from build123d import *

# Parameters (mm, degrees)
BOSS_EXTRUDE1_DEPTH = 3.175
SKETCH2_W           = 3.175
SKETCH2_H           = 6.992
SKETCH2_W_2         = 12.5
SKETCH2_H_2         = 3.175
SKETCH2_W_3         = 15
CUT_EXTRUDE1_DEPTH  = 4.1750001


with BuildPart() as part:
    # Sketch1 → Boss-Extrude1 (new body)
    with BuildSketch(Plane(origin=(0, 0, 0), x_dir=(1, 0, 0), z_dir=(0, 1, 0))):
        with BuildLine():
            add(Edge.make_bspline(
                [(0, 0), (2.315309036, 13.13077004), (22.407654518, 25), (42.5, 25)],
                knots=[0, 0, 0, 0, 0.5, 0.5, 0.5, 0.5], degree=3))
            Line((0, 0), (42.5, 0))
            Line((42.5, 0), (42.5, 25))
        make_face()
        with BuildLine():
            Line((42.5, 25), (42.5, 0))
            Line((42.5, 0), (85, 0))
            add(Edge.make_bspline(
                [(42.5, 25), (62.592345482, 25), (82.684690964, 13.13077004), (85, 0)],
                knots=[0.5, 0.5, 0.5, 0.5, 1, 1, 1, 1], degree=3))
        make_face()
    extrude(amount=BOSS_EXTRUDE1_DEPTH)

    # Sketch2 → Cut-Extrude1 (cut, through all)
    with BuildSketch(Plane.XZ):
        with Locations((64.0875, -11.504)):
            Rectangle(SKETCH2_W, SKETCH2_H)
        with Locations((20.9125, -11.504)):
            Rectangle(SKETCH2_W, SKETCH2_H)
        with Locations((78.75, -1.5875)):
            Rectangle(SKETCH2_W_2, SKETCH2_H_2)
        with Locations((6.25, -1.5875)):
            Rectangle(SKETCH2_W_2, SKETCH2_H_2)
        with Locations((42.5, -1.5875)):
            Rectangle(SKETCH2_W_3, SKETCH2_H_2)
    extrude(amount=-CUT_EXTRUDE1_DEPTH, mode=Mode.SUBTRACT)


solid = part.part
For this review, take the finished solid that the model builds, in its own axes (mm). A direction names the side the tool comes from. Give positions to 0.01 mm unless a question says otherwise; leave off trailing zeros. Answer as a JSON object with one key per item and string values. Group by question number.
Item 1: Wall thickness on line 1 along X through (y, z) = (0.9, -10.5) (3 decimals); line 2 along X through (y, z) = (2.25, -12) (3 decimals); line 3 along X through (y, z) = (2.05, -1.75): over which ranges is each line inside the solid? List them lowest first.
Item 2: Machinability: for faces 4 (the flat face through (64, 2, -15)), 5 (the flat face through (12.5, 2, -2)), 6 (the flat face through (35, 2, -2)), which of the approach directions +Z, -Z, +X, -X, +Y, -Y give a long, thin tool a straight path to every point of the face, cutting with its end or side? Answer none if there is none.
Item 3: Draft analysis for pull direction Z (two halves, no side actions). For faces 1 (the flat face through (21, 2, -15)), 2 (the flat face through (43, 0, -10)), 3 (the flat face through (42, 2, -3.175)), state which applies: pulls with the +Z half, pulls with the -Z half, needs draft (parallel to the pull), parting line crosses it, or undercut.
Item 4: Take a section at A-A on y = 2.55. Give the number of separate pieces and of enclosed holes in the cut face, and give its area (3 significant figures).
Item 5: Clearance check with flat-ended pins moving along their axes: pin 1 Ø1 at (x, y) = (21.5, 2.5) entering from -Z; pin 2 Ø1.6 at (x, y) = (64, 1.5) entering from -Z; pin 3 Ø1 at (y, z) = (1.5, -11) entering from +X. State where each tip first meets the part, or that it passes through.
Reported:
{
 "1": {"line 1": "5.736 to 19.325, 22.5 to 62.5, 65.675 to 79.264", "line 2": "7.239 to 19.325, 22.5 to 62.5, 65.675 to 77.761", "line 3": "12.5 to 35, 50 to 72.5"},
 "2": {"face 4": "+Y, -Y", "face 5": "+Z, -X, +Y, -Y", "face 6": "+Z, +Y, -Y"},
 "3": {"face 1": "undercut", "face 2": "needs draft", "face 3": "pulls with the +Z half"},
 "4": {"separate pieces": "1", "enclosed holes": "2", "area": "1,420 mm^2"},
 "5": {"pin 1": "z = -21.03", "pin 2": "z = -20.95", "pin 3": "x = 79.26"}
}
